Study the drawing (mm; zero at the part's minimum x, y, z) and answer. A direction names the side the tool comes from. Give positions to 0.01 mm unless a question says otherwise; leave off trailing zeros. Order: outer loops, then holes, each group sorted by start corner. A loop starts at its lowest first (then second) coordinate and runs counter-clockwise, first axis right, second up. Notation, with made-up numbers: (-33, 87.25) -> (23, 87.25) arc R32 ccw to (23, 121.25) -> close; hole circle Ø3 at (-0.5, 26.25). An arc over 180 degrees is marked (long way). Answer as CSV lines item,"result". Start each with the question number.
1. For the marked faces 1 and 2, determine the directions among +Z, -Z, +X, -X, +Y, -Y from which every point of the face is accessible in a straight line to the end or side of a thin tool.
2. A cutting plane is placed at D-D (z = 95). Give the vertices of the cut face in (x, y) (3 decimals), then the cut area to 3 significant figures.
3. A cutting plane is placed at B-B (y = 41.5). Give the vertices of the cut face in (x, z) (3 decimals), then the cut area to 3 significant figures.
4. Flat-ended cylindrical pins translate along their axes: pin 1 (5 mm diameter, centred on x = 14, z = 46.5, fed in from +Y) (3 decimals); pin 2 (5 mm diameter, centred on y = 33.5, z = 103.5, fed in from -X); pin 3 (12 mm diameter, centred on y = 10.5, z = 25.5, fed in from -X). Find the tip coordinate at first contact, or state that the pin passes through.
5. A cutting plane is placed at A-A (x = 6.35). State how many separate pieces and enclosed holes the cut face has, then the cut area to 3 significant figures.
6. Find the intervals of material crossed by L1, parallel to X at y = 1, z = 114 (1 decimal); L2, parallel to X at y = 2.35, z = 6.35; L3, parallel to Y at x = 41, z = 72 (3 decimals), in increasing order.
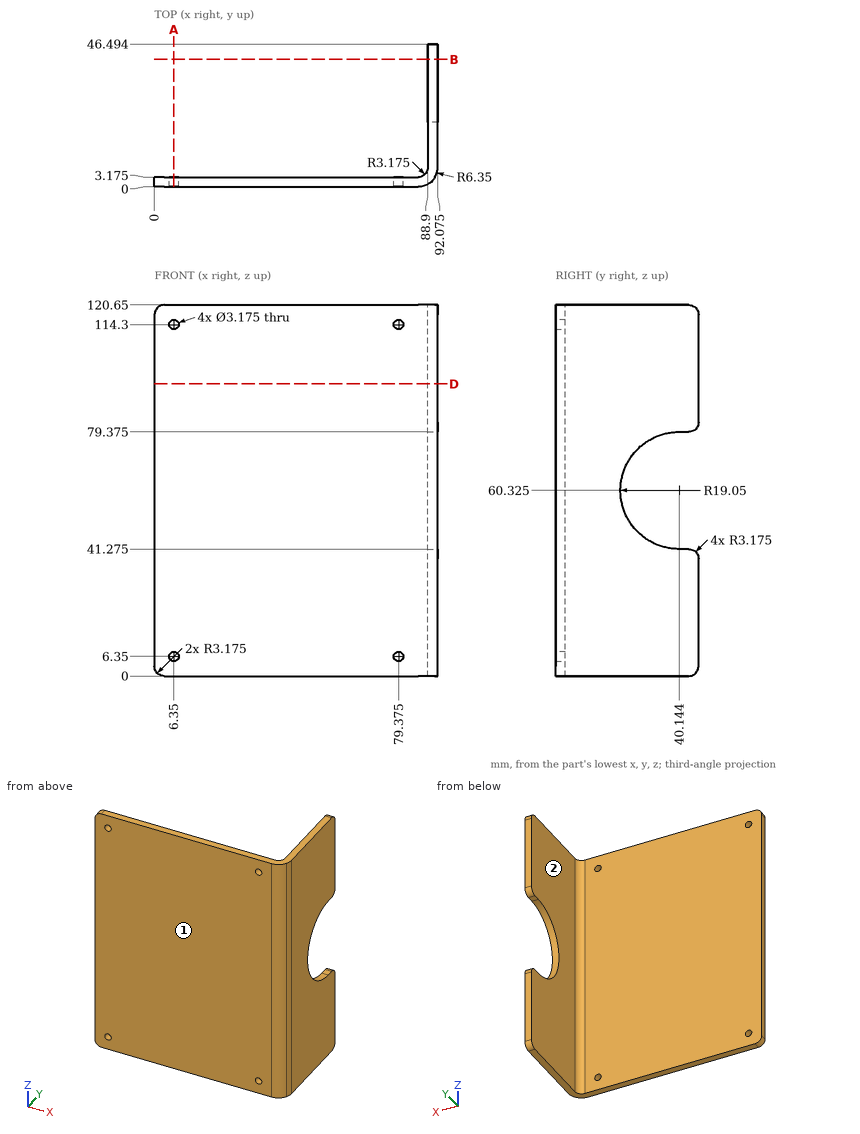
Answer sheet:
1,face 1,"+Z, -Z, +X, -X, -Y"
1,face 2,"+Z, -Z, -X, +Y"
2,outline,"(0, 0) -> (85.725, 0) arc R6.35 ccw to (92.075, 6.35) -> (92.075, 46.494) -> (88.9, 46.494) -> (88.9, 6.35) arc R3.175 cw to (85.725, 3.175) -> (0, 3.175) -> close"
2,area,"423 mm^2"
3,outline,"(88.9, 0) -> (92.075, 0) -> (92.075, 41.275) -> (88.9, 41.275) -> close; (88.9, 79.375) -> (92.075, 79.375) -> (92.075, 120.65) -> (88.9, 120.65) -> close"
3,area,"262 mm^2"
4,pin 1,"stops at y = 3.175"
4,pin 2,"stops at x = 88.9"
4,pin 3,"stops at x = 88.31"
5,separate pieces,"3"
5,enclosed holes,"0"
5,area,"363 mm^2"
6,L1,"x = 0 to 4.8, 7.9 to 77.8, 80.9 to 89.1"
6,L2,"x = 0 to 4.76, 7.94 to 77.79, 80.96 to 90.66"
6,L3,"y = 0 to 3.175"
